from build123d import *

# Parameters (mm, degrees)
SKETCH001_R     = 6
POCKET_DEPTH    = 8.820854
CHAMFER_SIZE    = 0.2
CHAMFER001_SIZE = 1


with BuildPart() as pocket:
    # Sketch003 → Revolution001 (revolve)
    with BuildSketch(Plane.XZ):
        Polygon((0, 1.180146), (5, 3), (5, 10), (0, 10), align=None)
    revolve(axis=Axis((0, 0, 0), (0, 0, 1)))

    # Sketch001 → Pocket (cut, through all)
    with BuildSketch(Plane(origin=(0, 0, 10), x_dir=(-1, 0, 0), z_dir=(0, 0, 1))):
        Circle(SKETCH001_R)
        Polygon((-1.443376, 2.5), (1.443376, 2.5), (2.886751, 0), (1.443376, -2.5), (-1.443376, -2.5), (-2.886751, 0), align=None, mode=Mode.SUBTRACT)
    extrude(amount=-POCKET_DEPTH, mode=Mode.SUBTRACT)


with BuildPart() as chamfer001:
    # Sketch → Revolution (revolve)
    with BuildSketch(Plane.XZ):
        Polygon((2.88675, 6), (5, 6), (5, 0), (3, 0), (3, -40), (0, -40), (0, 3.113247), align=None)
    revolve(axis=Axis((0, 0, 0), (0, 0, 1)))

    # Cut: cut Pocket
    add(pocket.part, mode=Mode.SUBTRACT)

    # Chamfer
    chamfer_edges = [chamfer001.edges().sort_by_distance(p)[0] for p in [
        (-5, 0, 6),
        (-5, 0, 0),
    ]]
    chamfer(chamfer_edges, length=CHAMFER_SIZE)

    # Chamfer001
    chamfer001_edges = [chamfer001.edges().sort_by_distance(p)[0] for p in [
        (-3, 0, -40),
    ]]
    chamfer(chamfer001_edges, length=CHAMFER001_SIZE)


solid = chamfer001.part
Work out the finished part from the listing and answer in its coordinate system (mm). A direction names the side the tool comes from. Give positions to 0.01 mm unless a question says otherwise; leave off trailing zeros. Loops run counter-clockwise (first coordinate to the right, second up) from the corner with the lowest first, then second, coordinate; pieces in that order, holes last. Notation, with made-up numbers: (-7, 74) - (39, 74) arc R28 cw to (39, 107) - close; hole circle Ø2 at (27.25, 69). An arc over 180 degrees is marked (long way). Answer in a Markdown table with one row per item.
(1) For a pull along X with two mould halves and no side action, classify faces 4 (the face through (-1.08, -4.88, 2.96)), 5 (the face through (0, 2.5, 4)), 6 (the face through (0, 0, -40)) as pulls with the +X half, pulls with the -X half, needs draft (parallel to the pull), parting line crosses it, or undercut.
Results list:
| item | result |
|---|---|
| face 4 | parting line crosses it |
| face 5 | undercut |
| face 6 | needs draft |
(2) Section A-A (z = -37) is taken. Give the vertices of the cut face in (x, y), and give its area (3 significant figures).
Results list:
| item | result |
|---|---|
| outline | circle Ø6 at (0, 0) |
| area | 28.3 mm² |
(3) Consider L1, parallel to Z at x = 1.5, y = 3; L2, parallel to Y at x = 0, z = -29; L3, parallel to Y at x = -2.5, z = -23.5. Determine where each line is inside the solid, lowest interval first. Write a range as [from, to].
Results list:
| item | result |
|---|---|
| L1 | z = [0, 6] |
| L2 | y = [-3, 3] |
| L3 | y = [-1.66, 1.66] |
(4) Flat-ended cylindrical pins translate along their axes: pin 1 Ø1.5 at (x, z) = (-3.5, -17.5) entering from -Y; pin 2 Ø4 at (x, y) = (2, 1.5) entering from -Z; pin 3 Ø5 at (y, z) = (-1, -6.5) entering from +X; pin 4 Ø3 at (x, z) = (2, -7.5) entering from -Y. Find the tip coordinate at first contact, or state that the pin passes through.
Results list:
| item | result |
|---|---|
| pin 1 | stops at y = -1.2 |
| pin 2 | stops at z = -40 |
| pin 3 | stops at x = 3 |
| pin 4 | stops at y = -2.96 |
(5) A tool of negligible diameter and unlimited length cuts with its end or side. For faces 1 (the face through (-2.175, 1.233, 4.072)), 2 (the face through (1, -3, 0)), 3 (the face through (0.1, -3.1, 6)), from which of +Z, -Z, +X, -X, +Y, -Y can it reach the whole face along a straight path? Write none if from no direction.
Results list:
| item | result |
|---|---|
| face 1 | +Z |
| face 2 | -Z |
| face 3 | +Z, +X, -X, +Y, -Y |
